Model file for the job. Use its own axes, mm. A direction names the side the tool comes from. Coordinates: 2 decimals unless noted, no trailing zeros. Order: outer loops, then holes, each group sorted by start corner. A loop starts at its lowest first (then second) coordinate and runs counter-clockwise, first axis right, second up.
from build123d import *

# Parameters (mm, degrees)
F1_DEPTH = 50


with BuildPart() as f1:
    # F0 (on Front) → F1 (new body, symmetric)
    with BuildSketch(Plane.XZ):
        Polygon((0, -14.5), (0, 14.5), (-5, 14.5), (-23, 32.5), (-32.5, 32.5), (-32.5, 10), (-27.5, 10), (-27.5, -10), (-32.5, -10), (-32.5, -32.5), (-23, -32.5), (-5, -14.5), align=None)
        Polygon((5, 14.5), (0, 14.5), (0, -14.5), (5, -14.5), (23, -32.5), (32.5, -32.5), (32.5, -10), (27.5, -10), (27.5, 10), (32.5, 10), (32.5, 32.5), (23, 32.5), align=None)
    extrude(amount=F1_DEPTH, both=True)


solid = f1.part
Q1. Cut at A-A, the plane z = -26. List the corners of the cut face in (x, y), plus the area to 3 significant figures.
Established:
outline: (-32.5, -50) - (-16.5, -50) - (-16.5, 50) - (-32.5, 50) - close; (16.5, -50) - (32.5, -50) - (32.5, 50) - (16.5, 50) - close
area: 3,200 mm2
Q2. Mould opens along X. For faces 1 (the face through (30, -1, 10)), 2 (the face through (-32.5, -1, 21)), 3 (the face through (-14.1, -0.7, -23.6)) say: pulls with the +X half, pulls with the -X half, needs draft (parallel to the pull), parting line crosses it, or undercut.
Established:
face 1: needs draft
face 2: pulls with the -X half
face 3: undercut
Q3. Cut at B-B, the plane z = 24. List the corners of the cut face in (x, y), plus the area to 3 significant figures.
Established:
outline: (-32.5, -50) - (-14.5, -50) - (-14.5, 50) - (-32.5, 50) - close; (14.5, -50) - (32.5, -50) - (32.5, 50) - (14.5, 50) - close
area: 3,600 mm2
Q4. Cut at C-C, the plane y = 18. List the corners of the cut face in (x, z).
Established:
outline: (-32.5, -32.5) - (-23, -32.5) - (-5, -14.5) - (5, -14.5) - (23, -32.5) - (32.5, -32.5) - (32.5, -10) - (27.5, -10) - (27.5, 10) - (32.5, 10) - (32.5, 32.5) - (23, 32.5) - (5, 14.5) - (-5, 14.5) - (-23, 32.5) - (-32.5, 32.5) - (-32.5, 10) - (-27.5, 10) - (-27.5, -10) - (-32.5, -10) - close
Q5. Probe line 1 (X direction, y = 21, z = -24); line 2 (Z direction, x = 29.5, y = -19); line 3 (X direction, y = -19, z = -23.5). List the from-to ranges inside material, lowest first.
Established:
line 1: x = -32.5 to -14.5, 14.5 to 32.5
line 2: z = -32.5 to -10, 10 to 32.5
line 3: x = -32.5 to -14, 14 to 32.5
Q6. Cut at D-D, the plane x = 2. List the corners of the cut face in (y, z).
Established:
outline: (-50, -14.5) - (50, -14.5) - (50, 14.5) - (-50, 14.5) - close
Q7. Drop flat-ended pins along their axis: P1, Ø3, axis at x = 0, y = -5.5, coming from the +Z side; P2, Ø6, axis at x = 2, z = -19.5, coming from the -Y side; P3, Ø1.5, axis at x = -15, y = -8, coming from the +Z side; P4, Ø8, axis at y = 7, z = 2.5, coming from the +X side. Give the stop position or say it passes through.
Established:
P1: stops at z = 14.5
P2: passes through
P3: stops at z = 25.25
P4: stops at x = 27.5
Q8. Which spindle directions (+Z, -Z, +X, -X, +Y, -Y) get a long thin tool onto all of the face, cutting with end or side? Do faces 4 (the face through (13.9, -0.7, -23.4)), 5 (the face through (-27.5, -1, 0)), 6 (the face through (30, -1, -10)). Say none if no direction does.
Established:
face 4: -Z, +Y, -Y
face 5: -X, +Y, -Y
face 6: +X, +Y, -Y
